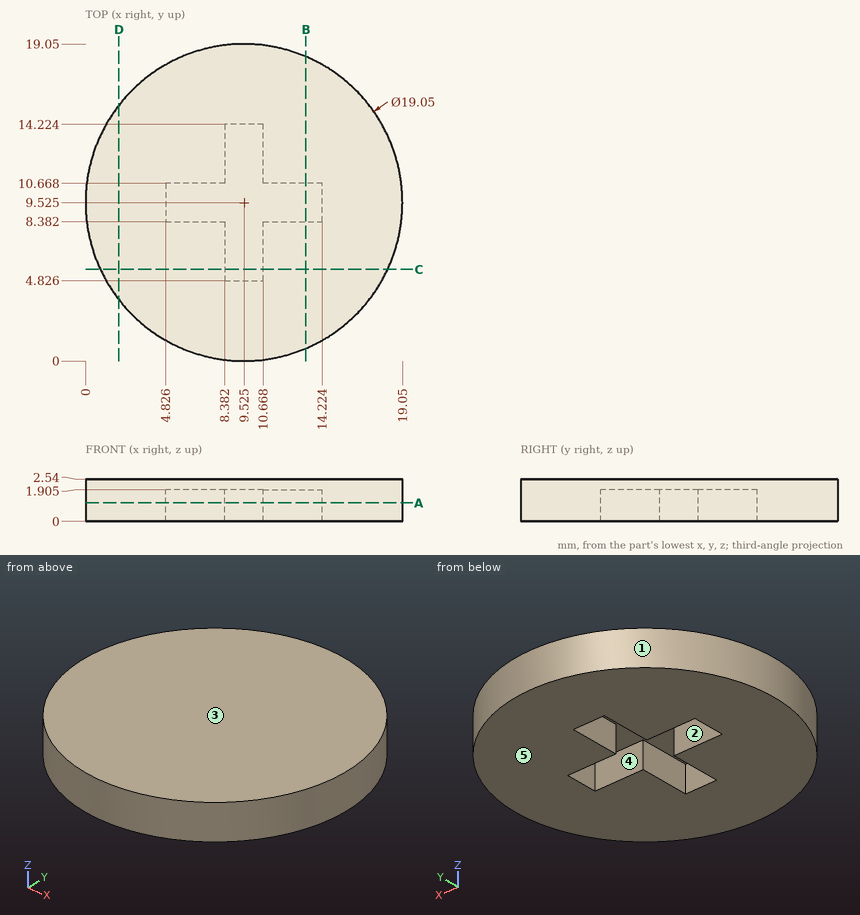
Print and shaded views of the part. All mm, measured from the part's lowest x, y and z. A direction names the side the tool comes from. Give positions to 0.01 mm unless a question says otherwise; leave off trailing zeros. Order: outer loops, then holes, each group sorted by start corner. A loop starts at its lowest first (then second) coordinate and runs counter-clockwise, first axis right, second up. Notation, with made-up numbers: (32, 89) - (43, 89) arc R8 ccw to (43, 93) - close; hole circle Ø5 at (-28, -22). An arc over 180 degrees is marked (long way). Use a Markdown table: item, result.
1) Saw through at C-C on y = 5.5. List the corners of the cut face in (x, z) (3 decimals).
Checked values:
| item | result |
|---|---|
| outline | (0.892, 0) - (8.382, 0) - (8.382, 1.905) - (10.668, 1.905) - (10.668, 0) - (18.158, 0) - (18.158, 2.54) - (0.892, 2.54) - close |
2) Probe L1, parallel to Z at x = 13.75, y = 10.25 (3 decimals); L2, parallel to X at y = 9, z = 0.2; L3, parallel to Y at x = 13.5, z = 0.9. List the from-to ranges inside material, lowest first. Write a range as from..to.
Checked values:
| item | result |
|---|---|
| L1 | 1.905..2.54 |
| L2 | 0.01..4.83, 14.22..19.04 |
| L3 | 0.87..8.38, 10.67..18.18 |
3) 3-axis set-ups, long thin cutter, end or side, ignore diameter. For the marked faces 4 and 5: which of +Z, -Z, +X, -X, +Y, -Y reach the whole face in a straight line?
Checked values:
| item | result |
|---|---|
| face 4 | -Z |
| face 5 | -Z, +X, -X, +Y, -Y |
4) Saw through at B-B on x = 13.25. List the corners of the cut face in (y, z) (3 decimals).
Checked values:
| item | result |
|---|---|
| outline | (0.759, 0) - (8.382, 0) - (8.382, 1.905) - (10.668, 1.905) - (10.668, 0) - (18.291, 0) - (18.291, 2.54) - (0.759, 2.54) - close |
5) Saw through at D-D on x = 2. List the corners of the cut face in (y, z).
Checked values:
| item | result |
|---|---|
| outline | (3.69, 0) - (15.36, 0) - (15.36, 2.54) - (3.69, 2.54) - close |
6) Flat gauge pins, fed straight in: P1, Ø3, axis at x = 9, y = 8.5, coming from the -Z side; P2, Ø0.6, axis at y = 13, z = 1.5, coming from the +X side; P3, Ø0.6, axis at y = 10, z = 1.5, coming from the -X side; P4, Ø0.6, axis at x = 6, z = 1, coming from the +Y side. Where does each tip first touch, or does it go through?
Checked values:
| item | result |
|---|---|
| P1 | z = 0 |
| P2 | x = 18.51 |
| P3 | x = 0 |
| P4 | y = 18.49 |
7) Saw through at A-A on z = 1.1. List the corners of the cut face in (x, y) (3 decimals).
Checked values:
| item | result |
|---|---|
| outline | circle Ø19.05 at (9.525, 9.525); hole (4.826, 8.382) - (8.382, 8.382) - (8.382, 4.826) - (10.668, 4.826) - (10.668, 8.382) - (14.224, 8.382) - (14.224, 10.668) - (10.668, 10.668) - (10.668, 14.224) - (8.382, 14.224) - (8.382, 10.668) - (4.826, 10.668) - close |
8) Two-plate mould, pull along Y, no slides. Class the marked faces 1, 2 and 3: +Y half, -Y half, draft (parallel to the pull), parting line (faces both ways), or undercut.
Checked values:
| item | result |
|---|---|
| face 1 | parting line |
| face 2 | undercut |
| face 3 | draft |
